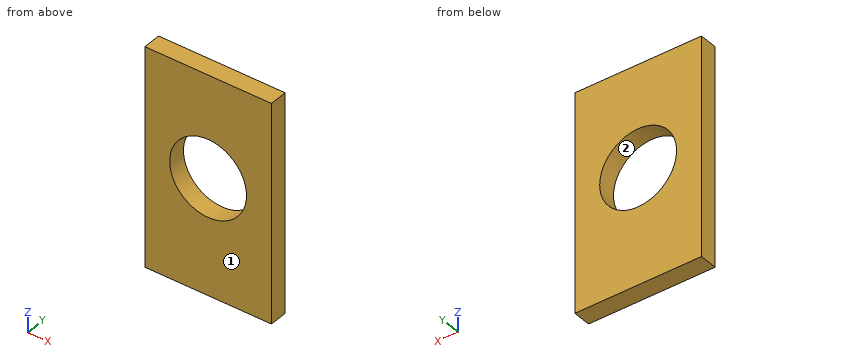
from build123d import *

# Parameters (mm, degrees)
CYLINDER881_R     = 8.5
CYLINDER881_DEPTH = 10
BOX425_W          = 28
BOX425_H          = 4
BOX425_DEPTH      = 48


with BuildPart() as obj1:
    # Cylinder881 → Cylinder881 (new body)
    with BuildSketch(Plane(origin=(44, 6, 51.5), x_dir=(1, 0, 0), z_dir=(0, -1, 0))):
        Circle(CYLINDER881_R)
    extrude(amount=CYLINDER881_DEPTH)


with BuildPart() as cut023:
    # Box425 → Box425 (new body)
    with BuildSketch(Plane(origin=(30, 0, 26), x_dir=(1, 0, 0), z_dir=(0, 0, 1))):
        with Locations((14, 2)):
            Rectangle(BOX425_W, BOX425_H)
    extrude(amount=BOX425_DEPTH)

    # Cut023: cut obj1
    add(obj1.part, mode=Mode.SUBTRACT)


solid = cut023.part
Input: part model. Units: mm. Frame: model coordinates. Face numbers are marked on the shaded views. Give positions to 0.01 mm unless a question says otherwise; leave off trailing zeros. Order: outer loops, then holes, each group sorted by start corner. A loop starts at its lowest first (then second) coordinate and runs counter-clockwise, first axis right, second up.
Q1. Draft query along Z for the marked faces 1 and 2. Return one class per face: +Z half, -Z half, draft (parallel to the pull), parting line (faces both ways), or undercut.
Checked values:
face 1: draft
face 2: undercut
Q2. Section B-B on x = 44. Output: boundary loops of the cut face in (y, z), and give its area (3 significant figures).
Checked values:
outline: (0, 26) - (4, 26) - (4, 43) - (0, 43) - close; (0, 60) - (4, 60) - (4, 74) - (0, 74) - close
area: 124 mm2
Q3. Section A-A on z = 51.5. Output: boundary loops of the cut face in (x, y).
Checked values:
outline: (30, 0) - (35.5, 0) - (35.5, 4) - (30, 4) - close; (52.5, 0) - (58, 0) - (58, 4) - (52.5, 4) - close
Q4. Section C-C on y = 3.1. Output: boundary loops of the cut face in (x, z).
Checked values:
outline: (30, 26) - (58, 26) - (58, 74) - (30, 74) - close; hole circle Ø17 at (44, 51.5)
Q5. Contact query for a flat-ended pin moving along its axis: pin 1 Ø3 at (x, z) = (34, 31.5) entering from -Y. Output: stop coordinate, or through.
Checked values:
pin 1: stops at y = 0
Q6. Ray query, probe 1 along Z at (x, y) = (44, 2.1); probe 2 along X at (y, z) = (2.5, 51.5); probe 3 along Z at (x, y) = (43, 0.25). Return the intervals inside material, ascending.
Checked values:
probe 1: z = 26 to 43, 60 to 74
probe 2: x = 30 to 35.5, 52.5 to 58
probe 3: z = 26 to 43.06, 59.94 to 74
